Read the model definition and answer for the solid it produces. Units are mm, in the model's axes. A direction names the side the tool comes from. Coordinates: 2 decimals unless noted, no trailing zeros. Loops run counter-clockwise (first coordinate to the right, second up) from the corner with the lowest first, then second, coordinate; pieces in that order, holes last.
from build123d import *

# Parameters (mm, degrees)
F0_W      = 20
F0_H      = 5
F0_H_2    = 3
F0_H_3    = 90
F0_H_4    = 34
F1_DEPTH  = 5
F2_W      = 20
F2_H      = 3
F2_H_2    = 5
F2_H_3    = 34
F3_DEPTH  = 5
F4_W      = 20
F4_H      = 3
F5_DEPTH  = 10
F6_R      = 2.5
F7_DEPTH  = 56
F8_R      = 5
F10_DEPTH = 5
F12_DEPTH = 5
F13_W     = 14
F13_H     = 84
F13_W_2   = 13.5
F13_H_2   = 28
F14_DEPTH = 2


with BuildPart() as f1:
    # F0 (on Top) → F1 (new body)
    with BuildSketch(Plane.XY):
        with Locations((0, 65)):
            Rectangle(F0_W, F0_H)
        with Locations((0, 61)):
            Rectangle(F0_W, F0_H_2)
        with Locations((0, 73)):
            Rectangle(F0_W, F0_H)
        with Locations((0, 20)):
            Rectangle(F0_W, F0_H)
        with Locations((0, 24)):
            Rectangle(F0_W, F0_H_2)
        with Locations((0, -30.5)):
            Rectangle(F0_W, F0_H_3)
        with Locations((0, 16)):
            Rectangle(F0_W, F0_H_2)
        with Locations((0, 69)):
            Rectangle(F0_W, F0_H_2)
        with Locations((0, 42.5)):
            Rectangle(F0_W, F0_H_4)
    extrude(amount=F1_DEPTH)

    # F2 (on Top) → F3 (join, through all)
    with BuildSketch(Plane.XY):
        with Locations((0, 69)):
            Rectangle(F2_W, F2_H)
        with Locations((0, 73)):
            Rectangle(F2_W, F2_H_2)
        with Locations((0, 65)):
            Rectangle(F2_W, F2_H_2)
        with Locations((0, 61)):
            Rectangle(F2_W, F2_H)
        with Locations((0, 24)):
            Rectangle(F2_W, F2_H)
        with Locations((0, 42.5)):
            Rectangle(F2_W, F2_H_3)
        with Locations((0, 20)):
            Rectangle(F2_W, F2_H_2)
        with Locations((0, 16)):
            Rectangle(F2_W, F2_H)
    extrude(amount=F3_DEPTH)

    # F4 (on face) → F5 (join)
    with BuildSketch(Plane.XY.offset(5)):
        with Locations((0, 69)):
            Rectangle(F4_W, F4_H)
        with Locations((0, 61)):
            Rectangle(F4_W, F4_H)
        with Locations((0, 24)):
            Rectangle(F4_W, F4_H)
        with Locations((0, 16)):
            Rectangle(F4_W, F4_H)
    extrude(amount=F5_DEPTH)

    # F6 (on face) → F7 (cut, through all)
    with BuildSketch(Plane.XZ.offset(-14.5)):
        with Locations((0, 10)):
            Circle(F6_R)
    extrude(amount=-F7_DEPTH, mode=Mode.SUBTRACT)

    # F8
    f8_edges = [f1.edges().sort_by_distance(p)[0] for p in [
        (10, 69, 15),
        (10, 61, 15),
        (-10, 61, 15),
        (-10, 69, 15),
        (10, 24, 15),
        (-10, 24, 15),
        (-10, 16, 15),
        (10, 16, 15),
    ]]
    fillet(f8_edges, radius=F8_R)

    # F9 (on face) → F10 (cut, through all)
    with BuildSketch(Plane.XY.offset(5)):
        Polygon((4.4243959922, 11.5), (-4.4243959922, 11.5), (0, 7.5180436071), align=None)
        Polygon((-2.2422706745, 5.5), (-7, 9.7819563929), (-7, 1.2180436071), align=None)
        Polygon((0, -14.5180436071), (-7, -20.8180436071), (-7, -22.1819563929), (0, -28.4819563929), (7, -22.1819563929), (7, -20.8180436071), align=None)
        Polygon((0, -32.5180436071), (-7, -38.8180436071), (-7, -40.1819563929), (0, -46.4819563929), (7, -40.1819563929), (7, -38.8180436071), align=None)
        Polygon((7, -52.7819563929), (7, -44.2180436071), (2.2422706745, -48.5), align=None)
        Polygon((-2.2422706745, -66.5), (-7, -62.2180436071), (-7, -70.7819563929), align=None)
        Polygon((7, -2.8180436071), (0, 3.4819563929), (-7, -2.8180436071), (-7, -4.1819563929), (0, -10.4819563929), (7, -4.1819563929), align=None)
        Polygon((7, 1.2180436071), (7, 9.7819563929), (2.2422706745, 5.5), align=None)
        Polygon((7, -16.7819563929), (7, -8.2180436071), (2.2422706745, -12.5), align=None)
        Polygon((-2.2422706745, -12.5), (-7, -8.2180436071), (-7, -16.7819563929), align=None)
        Polygon((7, -34.7819563929), (7, -26.2180436071), (2.2422706745, -30.5), align=None)
        Polygon((-2.2422706745, -30.5), (-7, -26.2180436071), (-7, -34.7819563929), align=None)
        Polygon((-2.2422706745, -48.5), (-7, -44.2180436071), (-7, -52.7819563929), align=None)
        Polygon((0, -50.5180436071), (-7, -56.8180436071), (-7, -58.1819563929), (0, -64.4819563929), (7, -58.1819563929), (7, -56.8180436071), align=None)
        Polygon((7, -70.7819563929), (7, -62.2180436071), (2.2422706745, -66.5), align=None)
        Polygon((4.4243959922, -72.5), (0, -68.5180436071), (-4.4243959922, -72.5), align=None)
    extrude(amount=-F10_DEPTH, mode=Mode.SUBTRACT)

    # F11 (on face) → F12 (cut, through all)
    with BuildSketch(Plane.XY.offset(5)):
        Polygon((-0.1457620642, 45.2106669293), (6.495022095, 56.5), (-7, 56.5), align=None)
        Polygon((6.5, 34.2647058824), (6.5, 50.7597279774), (1.5, 42.5), align=None)
        Polygon((6.5, 28.5), (-0.1468471232, 39.7794981484), (-6.9748553696, 28.5), align=None)
        Polygon((-1.7451316723, 42.4917385955), (-7, 51.4090909091), (-7, 33.5584624385), align=None)
    extrude(amount=-F12_DEPTH, mode=Mode.SUBTRACT)

    # F13 (on face) → F14 (cut, through all)
    with BuildSketch(Plane.XY.offset(5)):
        with Locations((0, -30.5)):
            Rectangle(F13_W, F13_H)
        with Locations((-0.25, 42.5)):
            Rectangle(F13_W_2, F13_H_2)
    extrude(amount=-F14_DEPTH, mode=Mode.SUBTRACT)


solid = f1.part
Item 1: A cutting plane is placed at A-A on z = 11.25. Give the number of separate pieces and of enclosed holes in the cut face, then the cut area to 3 significant figures.
Numbers:
separate pieces: 8
enclosed holes: 0
area: 184 mm2
Item 2: Find the intervals of material crossed by line 1 along Y through (x, z) = (-0.75, 6.75); line 2 along Z through (x, y) = (0, 24.25); line 3 along X through (y, z) = (35, 3.5), in increasing order.
Numbers:
line 1: y = 14.5 to 17.5, 22.5 to 25.5, 59.5 to 62.5, 67.5 to 70.5
line 2: z = 0 to 7.5, 12.5 to 15
line 3: x = -10 to -7, 6.5 to 10
Item 3: Given pin 1 (4 mm diameter, centred on y = 6.5, z = 8, fed in from +X) (3 decimals); pin 2 (3 mm diameter, centred on x = 0, y = -48, fed in from -Z); pin 3 (2.5 mm diameter, centred on x = 3, y = 20, fed in from +Z); pin 4 (8 mm diameter, centred on x = 0, z = 10, fed in from +Y), each flat-ended and moving along its own axis, determine where each tip first touches the part or whether it passes through.
Numbers:
pin 1: passes through
pin 2: stops at z = 0
pin 3: stops at z = 5
pin 4: stops at y = 70.5
Item 4: A cutting plane is placed at B-B on x = 8.5. Determine the outline of the cut face in (y, z), then the cut area to 3 significant figures.
Numbers:
outline: (-75.5, 0) - (75.5, 0) - (75.5, 5) - (70.5, 5) - (70.5, 13.57) - (67.5, 13.57) - (67.5, 5) - (62.5, 5) - (62.5, 13.57) - (59.5, 13.57) - (59.5, 5) - (25.5, 5) - (25.5, 13.57) - (22.5, 13.57) - (22.5, 5) - (17.5, 5) - (17.5, 13.57) - (14.5, 13.57) - (14.5, 5) - (-75.5, 5) - close
area: 858 mm2
Item 5: Determine the mould class of faces 6 (the face through (0, 73, 5)), 7 (the face through (0, 28.5, 3)), 8 (the face through (-9, 24, 13)), 9 (the face through (0, -72.5, 3)) for opening direction X: released by +X, released by -X, zero draft, split by the parting line, or undercut.
Numbers:
face 6: zero draft
face 7: undercut
face 8: released by -X
face 9: undercut
Item 6: Which of the six approach directions +Z, -Z, +X, -X, +Y, -Y give full straight-line access (tool end or side, diameter ignored) to faces 1 (the face through (0, -48, 3)), 2 (the face through (-3.549, -43.288, 1.521)), 3 (the face through (-2.4, 17.5, 8.8)), 4 (the face through (-2.4, 70.5, 8.8)), 5 (the face through (-0.54, 15.98, 7.56))?
Numbers:
face 1: +Z
face 2: +Z, -Z
face 3: +Z, +X, -X
face 4: +Z, +X, -X, +Y
face 5: +Y, -Y
